```python
from build123d import *

# Parameters (mm, degrees)
SKETCH_1_W      = 29.03316099
SKETCH_1_H      = 6.688317385
FILLET_1_R      = 3
SKETCH_2_R      = 4
EXTRUDE_1_DEPTH = 5
SHELL_1_T       = -2


with BuildPart() as part:
    # 草图1 → 旋转1 (revolve)
    with BuildSketch(Plane.XY, mode=Mode.PRIVATE) as revolve_1_sk:
        with Locations((14.516580495, 3.344158693)):
            Rectangle(SKETCH_1_W, SKETCH_1_H)
    revolve(revolve_1_sk.sketch.rotate(Axis((0, 6.688317385, 0), (0, -1, 0)), 90), axis=Axis((0, 6.688317385, 0), (0, -1, 0)))

    # 圆角1
    fillet_1_edges = [part.edges().sort_by_distance(p)[0] for p in [
        (0, 6.688317385, -29.03316099),
    ]]
    fillet(fillet_1_edges, radius=FILLET_1_R)

    # 草图2 → 凸台-拉伸1 (add)
    with BuildSketch(Plane(origin=(0, 6.688317385, 0), x_dir=(1, 0, 0), z_dir=(0, 1, 0))):
        with Locations(Location((-11.747239152, 8.851672142, 0), (0, 0, 90))):
            Circle(SKETCH_2_R)
    extrude(amount=EXTRUDE_1_DEPTH)

    # 抽壳1
    shell_1_openings = [part.faces().sort_by_distance(p)[0] for p in [
        (0, 0, 0),
    ]]
    offset(amount=SHELL_1_T, openings=shell_1_openings, kind=Kind.INTERSECTION)


solid = part.part
```
The listing builds one solid part. Answer for the finished solid, in the listing's coordinates (mm). A direction names the side the tool comes from. Coordinates: 2 decimals unless noted, no trailing zeros. Loops run counter-clockwise (first coordinate to the right, second up) from the corner with the lowest first, then second, coordinate; pieces in that order, holes last. Notation, with made-up numbers: M 2,44.5 L 37,44.5 A20 cw 37,57.5 Z; hole C 45,-32.75 d10. An arc over 180 degrees is marked long. Answer as CSV lines item,"result". Start each with the question number.
(1) Given pin 1 (5 mm diameter, centred on y = 8.5, z = 4, fed in from -X); pin 2 (15.5 mm diameter, centred on x = 2, z = -12, fed in from -Y); pin 3 (4 mm diameter, centred on x = 7.5, z = -11.5, fed in from +Y), each flat-ended and moving along its own axis, determine where each tip first touches the part or whether it passes through.
(2) The part is cut by section C-C (y = 5.75). Give the vertices of the cut face in (x, z), and give its area (3 significant figures).
(3) The part is cut by section D-D (y = 1). Give the vertices of the cut face in (x, z).
(4) The mould has two halves that part along X. Classify faces 4 (the cylindrical face through (-13.73, 7.15, -8.59)), 5 (the cylindrical face through (17.666, 1.87, -23.04)), 6 (the flat face through (-12, 9.688, -9)), 7 (the flat face through (-13, 0, 24)): pulls with the +X half, pulls with the -X half, needs draft (parallel to the pull), parting line crosses it, or undercut.
(5) The part is cut by section A-A (x = 0). Give the vertices of the cut face in (y, z), and give its area (3 significant figures).
(6) For faces 1 (the flat face through (-12, 11.688, -9)), 2 (the cylindrical face through (23.983, 1.87, 12.474)), 3 (the cylindrical face through (-8.2, 9.2, -10.7)), determine the directions among +Z, -Z, +X, -X, +Y, -Y from which every point of the face is accessible in a straight line to the end or side of a thin tool.
(7) Find the intervals of material crossed by L1, parallel to X at y = 2, z = 0; L2, parallel to Y at x = -14.5, z = 11.5; L3, parallel to X at y = 2.5, z = -24.5, in increasing order. Write a range as [from, to].
(8) The part is cut by section B-B (z = 0). Give the vertices of the cut face in (x, y), and give its area (3 significant figures).
Determined:
1,pin 1,"x = -27.68"
1,pin 2,"y = 4.69"
1,pin 3,"y = 6.69"
2,outline,"C 0,0 d56.42; hole C -11.75,-8.85 d4"
2,area,"2,490 mm2"
3,outline,"C 0,0 d58.07; hole C 0,0 d54.07"
4,face 4,"undercut"
4,face 5,"parting line crosses it"
4,face 6,"undercut"
4,face 7,"needs draft"
5,outline,"M 0,-29.03 L 3.69,-29.03 A3 ccw 6.69,-26.03 L 6.69,26.03 A3 ccw 3.69,29.03 L 0,29.03 L 0,27.03 L 3.69,27.03 A1 cw 4.69,26.03 L 4.69,-26.03 A1 cw 3.69,-27.03 L 0,-27.03 Z"
5,area,"131 mm2"
6,face 1,"+Z, -Z, +X, -X, +Y"
6,face 2,"-Y"
6,face 3,"+Y"
7,L1,"[-29.03, -27.03], [27.03, 29.03]"
7,L2,"[4.69, 6.69]"
7,L3,"[-15.58, -11.43], [11.43, 15.58]"
8,outline,"M -29.03,0 L -27.03,0 L -27.03,3.69 A1 cw -26.03,4.69 L 26.03,4.69 A1 cw 27.03,3.69 L 27.03,0 L 29.03,0 L 29.03,3.69 A3 ccw 26.03,6.69 L -26.03,6.69 A3 ccw -29.03,3.69 Z"
8,area,"131 mm2"
